from build123d import *

# Parameters (mm, degrees)
EXTRUDE_3_DEPTH     = 2
EXTRUDE_8_DEPTH     = 2
EXTRUDE_9_DEPTH     = 2
SKETCH_14_R         = 1.5
SKETCH_14_R_2       = 1
CUT_EXTRUDE_4_DEPTH = 72.399299806
SKETCH_15_R         = 1.5
SKETCH_15_R_2       = 1
CUT_EXTRUDE_5_DEPTH = 72.399299806
FILLET_9_R          = 1
FILLET_10_R         = 1
FILLET_11_R         = 1
FILLET_12_R         = 1


with BuildPart() as part:
    # 草图1 → 凸台-拉伸3 (new body)
    with BuildSketch(Plane.XY):
        with BuildLine():
            Line((-11.196428571, 28.5), (11.196428571, 28.5))
            ThreePointArc((11.196428571, 28.5), (16.264527304, 16.264527304), (28.5, 11.196428571))
            Line((28.5, 11.196428571), (28.5, -11.196428571))
            ThreePointArc((28.5, -11.196428571), (16.264527304, -16.264527304), (11.196428571, -28.5))
            Line((11.196428571, -28.5), (-11.196428571, -28.5))
            ThreePointArc((-11.196428571, -28.5), (-16.264527304, -16.264527304), (-28.5, -11.196428571))
            Line((-28.5, -11.196428571), (-28.5, 11.196428571))
            ThreePointArc((-28.5, 11.196428571), (-16.264527304, 16.264527304), (-11.196428571, 28.5))
        make_face()
    extrude(amount=EXTRUDE_3_DEPTH)

    # 草图12 → 凸台-拉伸8 (add)
    with BuildSketch(Plane(origin=(0, 28.5, 0), x_dir=(1, 0, 0), z_dir=(0, 1, 0))):
        with BuildLine():
            Line((-11.196428571, -2), (-11.196428571, 19))
            ThreePointArc((-11.196428571, 19), (0, 30.196428571), (11.196428571, 19))
            Line((11.196428571, 19), (11.196428571, -2))
            Line((11.196428571, -2), (-11.196428571, -2))
        make_face()
    extrude_8 = extrude(amount=-EXTRUDE_8_DEPTH)

    # 镜向6: 凸台-拉伸8 across plane
    add(extrude_8.mirror(Plane.ZX))

    # 草图13 → 凸台-拉伸9 (add)
    with BuildSketch(Plane(origin=(28.5, 0, 0), x_dir=(0, 0, -1), z_dir=(1, 0, 0))):
        with BuildLine():
            Line((0, 11.196428571), (-21, 11.196428571))
            ThreePointArc((-21, 11.196428571), (-32.196428571, 0), (-21, -11.196428571))
            Line((-21, -11.196428571), (0, -11.196428571))
            Line((0, -11.196428571), (0, 11.196428571))
        make_face()
    extrude_9 = extrude(amount=-EXTRUDE_9_DEPTH)

    # 镜向7: 凸台-拉伸9 across plane
    add(extrude_9.mirror(Plane(origin=(0, 0, 0), x_dir=(0, 0, 1), z_dir=(1, 0, 0))))

    # 草图14 → 切除-拉伸4 (cut, through all)
    with BuildSketch(Plane.ZY.offset(28.5)):
        with Locations((21, 0)):
            Circle(SKETCH_14_R)
        with Locations((21, 7)):
            Circle(SKETCH_14_R_2)
        with Locations((28, 0)):
            Circle(SKETCH_14_R_2)
        with Locations((21, -7)):
            Circle(SKETCH_14_R_2)
        with Locations((14, 0)):
            Circle(SKETCH_14_R_2)
    extrude(amount=-CUT_EXTRUDE_4_DEPTH, mode=Mode.SUBTRACT)

    # 草图15 → 切除-拉伸5 (cut, through all)
    with BuildSketch(Plane.XZ.offset(28.5)):
        with Locations(Location((0, -19, 0), (0, 0, 270))):
            Circle(SKETCH_15_R)
        with Locations(Location((0, -12, 0), (0, 0, 270))):
            Circle(SKETCH_15_R_2)
        with Locations(Location((7, -19, 0), (0, 0, 270))):
            Circle(SKETCH_15_R_2)
        with Locations(Location((0, -26, 0), (0, 0, 270))):
            Circle(SKETCH_15_R_2)
        with Locations(Location((-7, -19, 0), (0, 0, 270))):
            Circle(SKETCH_15_R_2)
    extrude(amount=-CUT_EXTRUDE_5_DEPTH, mode=Mode.SUBTRACT)

    # 圆角9
    fillet_9_edges = [part.edges().sort_by_distance(p)[0] for p in [
        (-28.5, 0, 0),
    ]]
    fillet(fillet_9_edges, radius=FILLET_9_R)

    # 圆角10
    fillet_10_edges = [part.edges().sort_by_distance(p)[0] for p in [
        (28.5, 0, 0),
    ]]
    fillet(fillet_10_edges, radius=FILLET_10_R)

    # 圆角11
    fillet_11_edges = [part.edges().sort_by_distance(p)[0] for p in [
        (0, -28.5, 2),
    ]]
    fillet(fillet_11_edges, radius=FILLET_11_R)

    # 圆角12
    fillet_12_edges = [part.edges().sort_by_distance(p)[0] for p in [
        (0, 28.5, 2),
    ]]
    fillet(fillet_12_edges, radius=FILLET_12_R)


solid = part.part
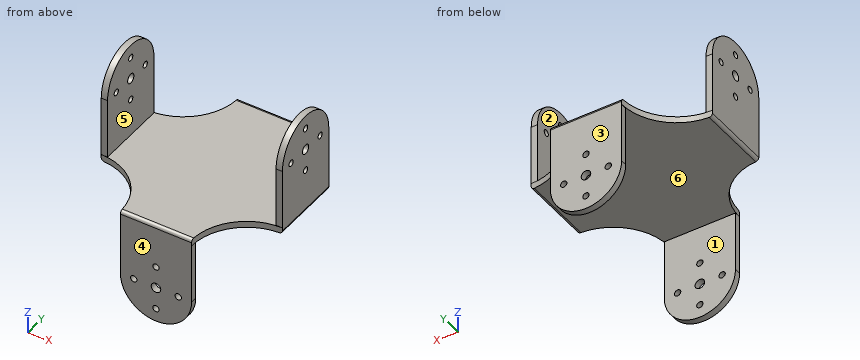
Could you check a few things on this model? Use its own coordinates, in mm. Face numbers are marked on the shaded views. A direction names the side the tool comes from. Coordinates: 2 decimals unless noted, no trailing zeros. Order: outer loops, then holes, each group sorted by start corner. A loop starts at its lowest first (then second) coordinate and runs counter-clockwise, first axis right, second up. Notation, with made-up numbers: (-17, 86.5) -> (5, 86.5) arc R31 cw to (5, 121.5) -> close; hole circle Ø11 at (31.5, 49.5). An arc over 180 degrees is marked (long way). One line per item, written item: value. Start each with the question number.
1) Imagine slicing it at B-B on y = 0. Count the separate pieces of the cut face and the enclosed holes in it, plus the area to 3 significant figures.
2) If I drill on L1, parallel to X at y = -27.3, z = -19; L2, parallel to Y at x = -6.5, z = -6, over which ranges is the centre line in solid material (lowest first)? Write a range as [from, to].
3) I'm going to push flat-ended pins straight in: pin 1 (2 mm diameter, centred on x = -27.5, z = 14, fed in from -Y); pin 2 (0.6 mm diameter, centred on y = -27.5, z = -5, fed in from +X); pin 3 (2 mm diameter, centred on y = 28, z = -6, fed in from -X). Where does each tip first touch, or does it pass through?
4) Which directions (+Z, -Z, +X, -X, +Y, -Y) give clear straight access to the entire face, cutting with the end or side of a thin tool? Please do the marked faces 4, 5 and 6.
5) Imagine slicing it at D-D on z = -12. List the corners of the cut face in (x, y) for me.
6) We'd pull the mould along Y, two halves only. Please class the marked faces 1, 2 and 3: +Y half, -Y half, draft (parallel to the pull), parting line (faces both ways), or undercut.
7) Imagine slicing it at A-A on z = 10. List the corners of the cut face in (x, y) for me, plus the area to 3 significant figures.
Answer list:
1. separate pieces: 7
1. enclosed holes: 0
1. area: 206 mm2
2. L1: x = [-11.2, -8], [-6, -1.5], [1.5, 6], [8, 11.2]
2. L2: y = [-28.5, -26.5], [26.5, 28.5]
3. pin 1: stops at y = -11.2
3. pin 2: stops at x = 11.2
3. pin 3: stops at x = -11.2
4. face 4: +Z, -Z, +X, -X, -Y
4. face 5: +Z, +Y, -Y
4. face 6: -Z, +X, -X
5. outline: (-11.2, -28.5) -> (-1, -28.5) -> (-1, -26.5) -> (-11.2, -26.5) -> close; (-11.2, 26.5) -> (-1, 26.5) -> (-1, 28.5) -> (-11.2, 28.5) -> close; (1, -28.5) -> (11.2, -28.5) -> (11.2, -26.5) -> (1, -26.5) -> close; (1, 26.5) -> (11.2, 26.5) -> (11.2, 28.5) -> (1, 28.5) -> close
6. face 1: undercut
6. face 2: draft
6. face 3: +Y half
7. outline: (-28.5, -11.2) -> (-26.5, -11.2) -> (-26.5, 11.2) -> (-28.5, 11.2) -> close; (26.5, -11.2) -> (28.5, -11.2) -> (28.5, 11.2) -> (26.5, 11.2) -> close
7. area: 89.6 mm2
